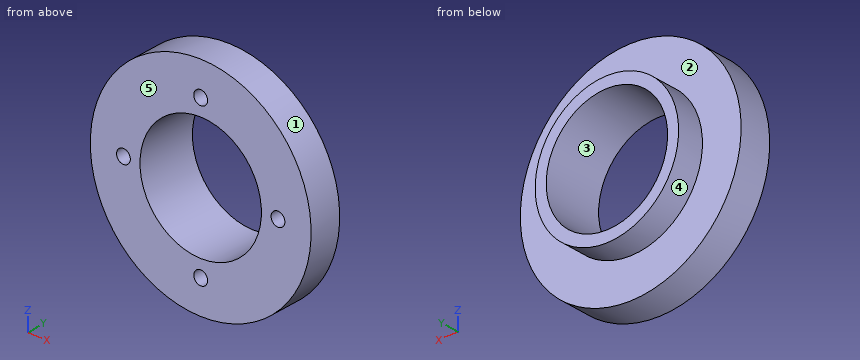
from build123d import *

# Parameters (mm, degrees)
SKETCH_1_R             = 20
SKETCH_1_R_2           = 11
EXTRUDE_1_DEPTH        = 6
SKETCH_2_R             = 13
SKETCH_2_R_2           = 11
EXTRUDE_2_DEPTH        = 5
HOLE_WIZARD_M3_1_D     = 2.5
HOLE_WIZARD_M3_1_DEPTH = 5
HOLE_WIZARD_M3_1_TIP   = 0.751075774


with BuildPart() as part:
    # 草图1 → 凸台-拉伸1 (new body)
    with BuildSketch(Plane(origin=(0, 0, 0), x_dir=(1, 0, 0), z_dir=(0, 1, 0))):
        with Locations(Location((0, 0, 0), (0, 0, 270))):
            Circle(SKETCH_1_R)
        with Locations(Location((0, 0, 0), (0, 0, 270))):
            Circle(SKETCH_1_R_2, mode=Mode.SUBTRACT)
    extrude(amount=EXTRUDE_1_DEPTH)

    # 草图2 → 凸台-拉伸2 (add)
    with BuildSketch(Plane(origin=(0, 6, 0), x_dir=(1, 0, 0), z_dir=(0, 1, 0))):
        with Locations(Location((0, 0, 0), (0, 0, 270))):
            Circle(SKETCH_2_R)
        with Locations(Location((0, 0, 0), (0, 0, 270))):
            Circle(SKETCH_2_R_2, mode=Mode.SUBTRACT)
    extrude(amount=EXTRUDE_2_DEPTH)

    # M3 螺纹孔1
    with Locations(Plane(origin=(0, 0, 0), x_dir=(-1, 0, 0), z_dir=(0, -1, 0))):
        with Locations((-14, 0), (0, -14), (14, 0), (0, 14)):
            Hole(HOLE_WIZARD_M3_1_D / 2, depth=HOLE_WIZARD_M3_1_DEPTH)
            with Locations((0, 0, -(HOLE_WIZARD_M3_1_DEPTH + HOLE_WIZARD_M3_1_TIP / 2))):  # 118° drill point
                Cone(0, HOLE_WIZARD_M3_1_D / 2, HOLE_WIZARD_M3_1_TIP, mode=Mode.SUBTRACT)


solid = part.part
Source: CAD feature listing. Evaluate the final solid. Frame: model axes, mm. Face numbers are marked on the shaded views. A direction names the side the tool comes from. Give positions to 0.01 mm unless a question says otherwise; leave off trailing zeros. Write each loop counter-clockwise with the first axis right and the second up, starting at its lowest first coordinate (ties: lowest second). Pieces come first, ordered by that corner, then holes. Notation, with made-up numbers: (81.25, 88.5) -> (90.25, 88.5) arc R18 cw to (90.25, 101.5) -> close; hole circle Ø5 at (46, -3.75). An arc over 180 degrees is marked (long way). Return JSON: item names as keys, results as strings. Group by question number.
1. Section B-B, the plane z = -4.5. Output: boundary loops of the cut face in (x, y).
2. Pin query (flat end, axial travel): pin 1 Ø1.5 at (x, y) = (10.5, 8.5) entering from +Z; pin 2 Ø2 at (x, z) = (0, -14) entering from -Y; pin 3 Ø2 at (x, y) = (-9, 3.5) entering from +Z. Return the tip coordinate at first contact, or that it passes through.
3. Access query for the marked faces 1 and 2. Directions: +Z, -Z, +X, -X, +Y, -Y. A direction counts if a zero-diameter tool reaches every point of the face in a straight line with its end or side. Return the directions, or none.
4. Section C-C, the plane y = 7. Output: boundary loops of the cut face in (x, z).
5. Mould query, pull axis X, two halves, no side actions, for the marked faces 3, 4 and 5. Classes: +X half, -X half, draft (parallel to the pull), parting line (faces both ways), or undercut.
6. Section A-A, the plane x = -3. Output: boundary loops of the cut face in (y, z).
7. Section D-D, the plane x = 16. Output: boundary loops of the cut face in (y, z).
8. Material intervals for line 1 (Y direction, x = -14.5, z = -1.5); line 2 (Z direction, x = 10, y = 8.75); line 3 (X direction, y = 3.25, z = -13), sorted ascending. Write a range as from..to.
Determined:
{
 "1": {"outline": "(-19.49, 0) -> (-10.04, 0) -> (-10.04, 11) -> (-12.2, 11) -> (-12.2, 6) -> (-19.49, 6) -> close; (10.04, 0) -> (19.49, 0) -> (19.49, 6) -> (12.2, 6) -> (12.2, 11) -> (10.04, 11) -> close"},
 "2": {"pin 1": "stops at z = 8.6", "pin 2": "stops at y = 5.15", "pin 3": "stops at z = 18.33"},
 "3": {"face 1": "+Y, -Y", "face 2": "+Y"},
 "4": {"outline": "circle Ø26 at (0, 0); hole circle Ø22 at (0, 0)"},
 "5": {"face 3": "undercut", "face 4": "parting line", "face 5": "draft"},
 "6": {"outline": "(0, -19.77) -> (6, -19.77) -> (6, -12.65) -> (11, -12.65) -> (11, -10.58) -> (0, -10.58) -> close; (0, 10.58) -> (11, 10.58) -> (11, 12.65) -> (6, 12.65) -> (6, 19.77) -> (0, 19.77) -> close"},
 "7": {"outline": "(0, -12) -> (6, -12) -> (6, 12) -> (0, 12) -> close"},
 "8": {"line 1": "y = 0..6", "line 2": "z = -8.31..-4.58, 4.58..8.31", "line 3": "x = -15.2..-0.75, 0.75..15.2"}
}
